The listing builds one solid part. Answer for the finished solid, in the listing's coordinates (mm). A direction names the side the tool comes from. Round coordinates to 2 decimals unless told otherwise and drop trailing zeros. Loops run counter-clockwise (first coordinate to the right, second up) from the corner with the lowest first, then second, coordinate; pieces in that order, holes last. Notation, with made-up numbers: (47.5, 68) - (63.5, 68) arc R4 cw to (63.5, 75) - close; hole circle Ø2 at (64, -22.5). An arc over 180 degrees is marked (long way). One line per question, with ' | ' between items. Start each with the question number.
from build123d import *

# Parameters (mm, degrees)
CROQUIS1_R                 = 10
SALIENTE_EXTRUIR1_DEPTH    = 25
CROQUIS3_R                 = 2.5
CORTAR_EXTRUIR2_DEPTH      = 52.961524227
CORTAR_EXTRUIR1_DEPTH      = 30
CORTAR_EXTRUIR3_REACH      = 39.417
CORTAR_EXTRUIR3_END_RADIUS = 2.5
CROQUIS7_R                 = 1.75


with BuildPart() as part:
    # Croquis1 → Saliente-Extruir1 (new, symmetric)
    with BuildSketch(Plane(origin=(0, 0, 0), x_dir=(1, 0, 0), z_dir=(0, 1, 0))):
        with Locations(Location((0, 0, 0), (0, 0, 270))):
            Circle(CROQUIS1_R)
    extrude(amount=SALIENTE_EXTRUIR1_DEPTH, both=True)

    # Croquis3 → Cortar-Extruir2 (cut, through all)
    with BuildSketch(Plane(origin=(0, 25, 0), x_dir=(1, 0, 0), z_dir=(0, 1, 0))):
        with Locations(Location((0, 0, 0), (0, 0, 270))):
            Circle(CROQUIS3_R)
    extrude(amount=-CORTAR_EXTRUIR2_DEPTH, mode=Mode.SUBTRACT)

    # Croquis2 → Cortar-Extruir1 (cut)
    with BuildSketch(Plane(origin=(0, 25, 0), x_dir=(1, 0, 0), z_dir=(0, 1, 0))):
        with BuildLine():
            Line((-7.141428429, 7), (7.141428429, 7))
            ThreePointArc((7.141428429, 7), (0, -10), (-7.141428429, 7))
        make_face()
    extrude(amount=-CORTAR_EXTRUIR1_DEPTH, mode=Mode.SUBTRACT)

    # Cortar-Extruir3: up to this cylinder (the profile starts outside it)
    cortar_extruir3_end = Plane(origin=(0, -10, 0), z_dir=(0, 1, 0)) * Cylinder(CORTAR_EXTRUIR3_END_RADIUS, 84.834, mode=Mode.PRIVATE)
    # Croquis7 → Cortar-Extruir3 (cut, up to the surface)
    with BuildSketch(Plane(origin=(0, -5, 10), x_dir=(1, 0, 0), z_dir=(0, 0, 1)), mode=Mode.PRIVATE) as cortar_extruir3_sk1:
        with Locations((0, -5)):
            Circle(CROQUIS7_R)
    cortar_extruir3_tool1 = extrude(cortar_extruir3_sk1.sketch, amount=-CORTAR_EXTRUIR3_REACH, mode=Mode.PRIVATE) - cortar_extruir3_end
    add(cortar_extruir3_tool1.solids().sort_by_distance((0, -10, 10))[0], mode=Mode.SUBTRACT)


solid = part.part
(1) Consider L1, parallel to Y at x = 0, z = 5.5; L2, parallel to Y at x = -6, z = 2.75; L3, parallel to X at y = -20, z = 0. Determine where each line is inside the solid, lowest interval first.
(2) Find section A-A on z = 0. Write down the section's boundary in (x, y), plus the area to 3 significant figures.
(3) Find section D-D on y = 14.5. Write down the section's boundary in (x, z).
(4) Determine the mould class of faces 1 (the flat face through (-2, -25, 2)), 2 (the cylindrical face through (0, -5, -10)), 3 (the cylindrical face through (0.1, -14.9, -2.5)) for opening direction X: pulls with the +X half, pulls with the -X half, needs draft (parallel to the pull), parting line crosses it, or undercut.
(5) A tool of negligible diameter and unlimited length cuts with its end or side. For faces 4 (the flat face through (2.4, -5, 1.4)), 5 (the cylindrical face through (-1.75, -9.92, 5.95)), 6 (the flat face through (0, 25, -8)), from which of +Z, -Z, +X, -X, +Y, -Y can it reach the whole face along a straight path? Write none if from no direction.
(6) Find section C-C on y = -14. Write down the section's boundary in (x, z).
(7) Find section B-B on x = 0. Write down the section's boundary in (y, z), plus the area to 3 significant figures.
(8) Each of these flat-tipped pins is pushed along its axis until it touches: P1, Ø4, axis at x = 2.5, y = -8.5, coming from the +Z side; P2, Ø10, axis at x = 7, y = -13, coming from the -Z side; P3, Ø3, axis at x = 0, y = -10, coming from the +Z side. Where does it stop, or does it pass through?
Answer below:
1) L1: -25 to -11.75, -8.25 to -5 | L2: -25 to -5 | L3: -10 to -2.5, 2.5 to 10
2) outline: (-10, -25) - (-2.5, -25) - (-2.5, -5) - (-10, -5) - close; (2.5, -25) - (10, -25) - (10, -5) - (2.5, -5) - close | area: 300 mm2
3) outline: (-7.14, -7) arc R10 ccw to (7.14, -7) - close
4) face 1: needs draft | face 2: parting line crosses it | face 3: undercut
5) face 4: +Z, +X, -X, +Y | face 5: +Z | face 6: +Z, -Z, +X, -X, +Y
6) outline: circle Ø20 at (0, 0); hole circle Ø5 at (0, 0)
7) outline: (-25, -10) - (25, -10) - (25, -7) - (-5, -7) - (-5, -2.5) - (-25, -2.5) - close; (-25, 2.5) - (-11.75, 2.5) - (-11.75, 10) - (-25, 10) - close; (-8.25, 2.5) - (-5, 2.5) - (-5, 10) - (-8.25, 10) - close | area: 364 mm2
8) P1: z = 9.99 | P2: z = -9.8 | P3: z = -2
